Source: three-view drawing plus pictorial views. Frame: mm from the lowest corner of the part. A direction names the side the tool comes from. Coordinates: 2 decimals unless noted, no trailing zeros. Order: outer loops, then holes, each group sorted by start corner. A loop starts at its lowest first (then second) coordinate and runs counter-clockwise, first axis right, second up. Notation, with made-up numbers: M -22.5,-31.75 L 28.5,-31.75 A20 ccw 28.5,-25.75 Z; hole C -29,16.5 d6. An arc over 180 degrees is marked long. Use CSV: the item, a comma, the result in double quotes. Start each with the question number.
Q1. Section query A-A, the plane z = 16.5. Output: boundary loops of the cut face in (x, y), and give its area (3 significant figures).
Q2. First-contact query: P1, Ø5, axis at x = 29.5, y = 6.5, coming from the +Z side; P2, Ø2.5, axis at x = 34.5, y = 16.5, coming from the +Z side; P3, Ø5, axis at x = 47.5, z = 11, coming from the -Y side. Flat tips, straight axial feed; report the tip coordinate or a pass-through.
Q3. Section query B-B, the plane x = 29. Output: boundary loops of the cut face in (y, z).
Q4. Ray query, probe 1 along Y at (x, z) = (47.5, 14.5); probe 2 along X at (y, z) = (15.5, 22.25); probe 3 along Z at (x, y) = (7.5, 3.5). Return the intervals inside material, ascending.
Q5. Access query for the marked faces 1 and 2. Directions: +Z, -Z, +X, -X, +Y, -Y. A direction counts if a zero-diameter tool reaches every point of the face in a straight line with its end or side. Return the directions, or none.
Q6. Section query D-D, the plane z = 6. Output: boundary loops of the cut face in (x, y), and give its area (3 significant figures).
Q7. Section query C-C, the plane y = 6. Output: boundary loops of the cut face in (x, z).
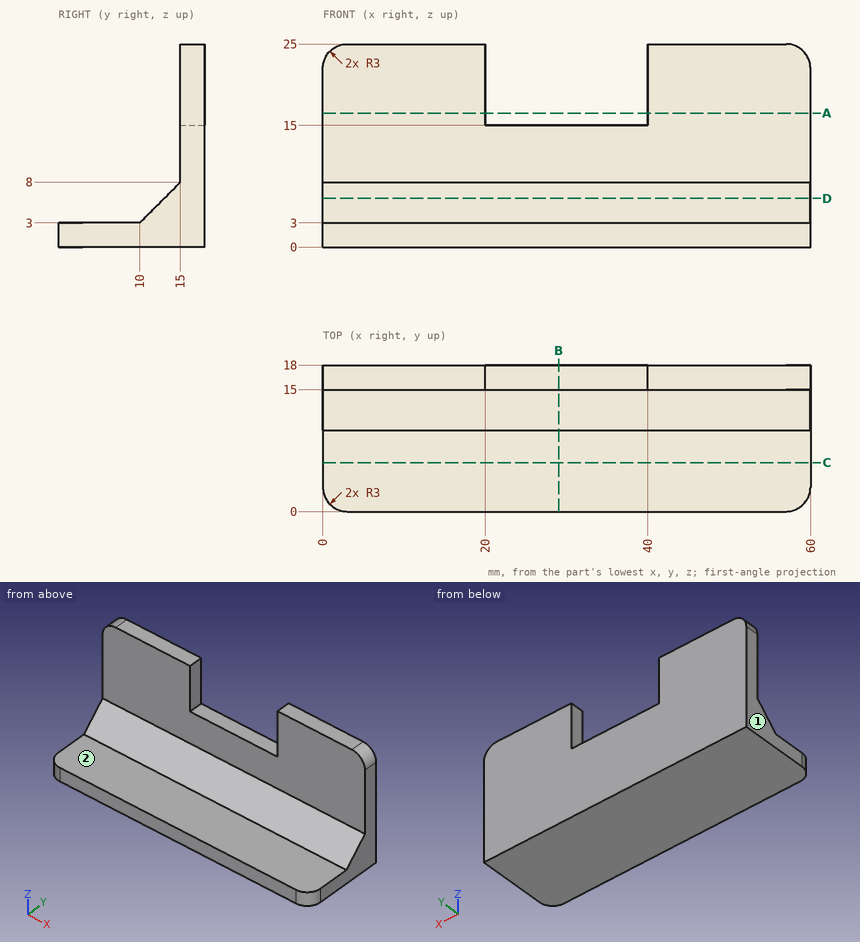
Responses:
1,outline,"M 0,15 L 20,15 L 20,18 L 0,18 Z; M 40,15 L 60,15 L 60,18 L 40,18 Z"
1,area,"120 mm²"
2,P1,"stops at z = 3"
2,P2,"stops at z = 15"
2,P3,"stops at y = 15"
3,outline,"M 0,0 L 18,0 L 18,15 L 15,15 L 15,8 L 10,3 L 0,3 Z"
4,probe 1,"y = 15 to 18"
4,probe 2,"x = 0.01 to 20, 40 to 59.99"
4,probe 3,"z = 0 to 3"
5,face 1,"+Z, -Z, -X, +Y, -Y"
5,face 2,"+Z, +X, -X, -Y"
6,outline,"M 0,13 L 60,13 L 60,18 L 0,18 Z"
6,area,"300 mm²"
7,outline,"M 0,0 L 60,0 L 60,3 L 0,3 Z"
